from build123d import *


with BuildPart() as part:
    # Croquis1 → Revolución3 (revolve)
    with BuildSketch(Plane.XY, mode=Mode.PRIVATE) as revoluci_n3_sk:
        with BuildLine():
            Line((0, 0), (15, 0))
            Line((15, 0), (15, 3))
            Line((15, 3), (13, 5))
            ThreePointArc((13, 5), (14.274991786, 10.413090898), (10, 13.97))
            Line((10, 13.97), (10, 14.97))
            ThreePointArc((10, 14.97), (9.414213562, 16.384213562), (8, 16.97))
            ThreePointArc((8, 16.97), (5.752892651, 28.90684447), (5, 41.03))
            ThreePointArc((5, 41.03), (6.794268653, 42.179508288), (6.5, 44.29))
            ThreePointArc((6.5, 44.29), (8.500795551, 54.317512481), (0, 60))
            Line((0, 60), (0, 0))
        make_face()
    revolve(revoluci_n3_sk.sketch.rotate(Axis((0, 60, 0), (0, -1, 0)), 90), axis=Axis((0, 60, 0), (0, -1, 0)))


solid = part.part
The listing builds one solid part. Answer for the finished solid, in the listing's coordinates (mm). A direction names the side the tool comes from. Coordinates: 2 decimals unless noted, no trailing zeros. Order: outer loops, then holes, each group sorted by start corner. A loop starts at its lowest first (then second) coordinate and runs counter-clockwise, first axis right, second up.
Q1. Given P1, Ø6, axis at x = 11, y = 40, coming from the +Z side; P2, Ø12, axis at y = 9.5, z = -11, coming from the +X side; P3, Ø3, axis at y = 24, z = -4, coming from the -X side; P4, Ø2, axis at y = 21, z = 4.5, coming from the +X side, each flat-ended and moving along its own axis, determine where each tip first touches the part or whether it passes through.
Q2. A cutting plane is placed at C-C, the plane y = 4. Write down the section's boundary in (x, z), and give its area (3 significant figures).
Q3. Which of the six approach directions +Z, -Z, +X, -X, +Y, -Y give full straight-line access (tool end or side, diameter ignored) to faces 1 (the face through (-0.44, 14.48, -9.99)), 2 (the face through (-12.65, 1.52, 8.06))?
Q4. Consider line 1 (Y direction, x = -11.75, z = 6); line 2 (Y direction, x = 7.5, z = 11); line 3 (X direction, y = 6, z = 9.5). Determine where each line is inside the solid, lowest interval first.
Q5. A cutting plane is placed at D-D, the plane y = 12.5. Write down the section's boundary in (x, z), and give its area (3 significant figures).
Q6. A cutting plane is placed at B-B, the plane x = 0. Write down the section's boundary in (y, z).
Q7. A cutting plane is placed at A-A, the plane z = 0. Write down the section's boundary in (x, y), and give its area (3 significant figures).
Answers follow:
1. P1: passes through
1. P2: stops at x = 13.65
1. P3: stops at x = -6.05
1. P4: stops at x = 6.19
2. outline: circle Ø28 at (0, 0)
2. area: 616 mm2
3. face 1: +Y
3. face 2: +Y, -Y
4. line 1: y = 0 to 4.81, 5.2 to 12.27
4. line 2: y = 0 to 4.69, 5.34 to 12.13
4. line 3: x = -9.99 to 9.99
5. outline: circle Ø25.95 at (0, 0)
5. area: 529 mm2
6. outline: (0, -15) - (3, -15) - (5, -13) arc R5.28 ccw to (13.97, -10) - (14.97, -10) arc R2 ccw to (16.97, -8) arc R97.98 cw to (41.03, -5) arc R1.98 ccw to (44.29, -6.5) arc R9.2 ccw (long way) to (44.29, 6.5) arc R1.98 ccw to (41.03, 5) arc R97.98 cw to (16.97, 8) arc R2 ccw to (14.97, 10) - (13.97, 10) arc R5.28 ccw to (5, 13) - (3, 15) - (0, 15) - close
7. outline: (-15, 0) - (15, 0) - (15, 3) - (13, 5) arc R5.28 ccw to (10, 13.97) - (10, 14.97) arc R2 ccw to (8, 16.97) arc R97.98 cw to (5, 41.03) arc R1.98 ccw to (6.5, 44.29) arc R9.2 ccw (long way) to (-6.5, 44.29) arc R1.98 ccw to (-5, 41.03) arc R97.98 cw to (-8, 16.97) arc R2 ccw to (-10, 14.97) - (-10, 13.97) arc R5.28 ccw to (-13, 5) - (-15, 3) - close
7. area: 1,020 mm2
